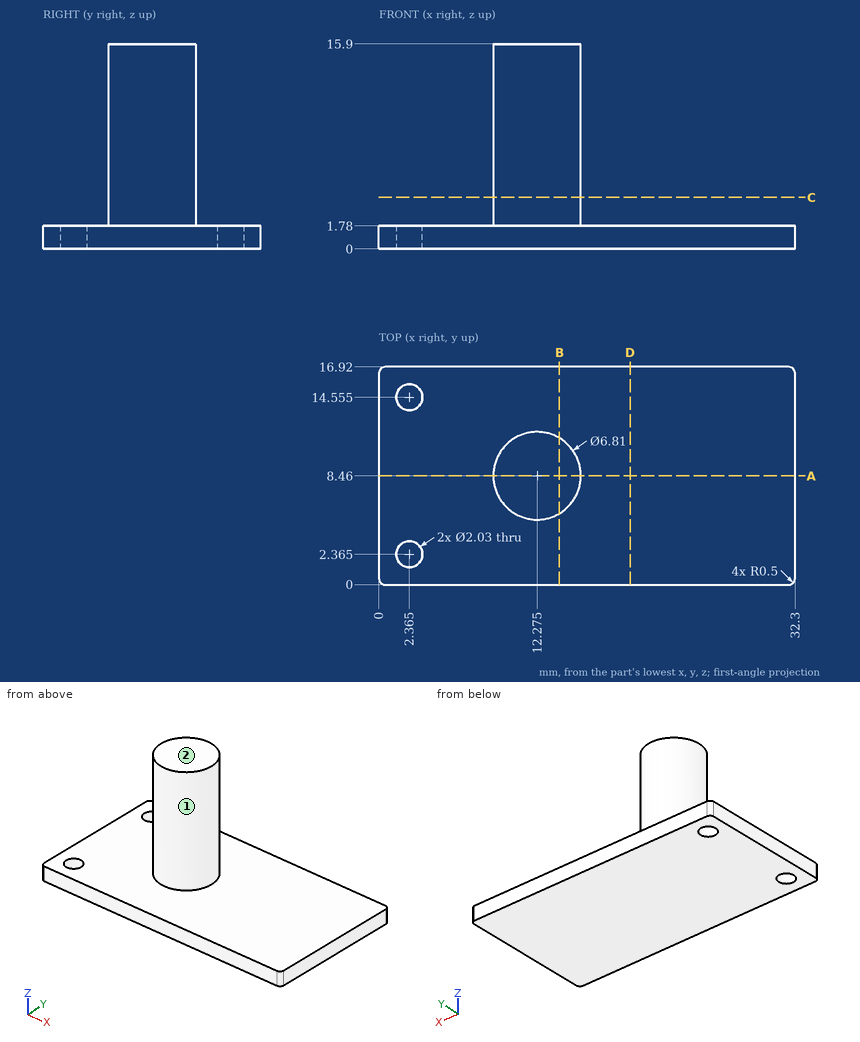
Answer from the drawing. Dimensions are ordinates in mm from the lowest x, y and z of the part. A direction names the side the tool comes from. Give positions to 0.01 mm unless a question says otherwise; leave off trailing zeros. Loops run counter-clockwise (first coordinate to the right, second up) from the corner with the lowest first, then second, coordinate; pieces in that order, holes last. Notation, with made-up numbers: (42.25, 55) - (57.25, 55) arc R25 ccw to (57.25, 78) - close; hole circle Ø8 at (55, 55.5). An arc over 180 degrees is marked (long way). Answer as a JSON object with one key per item and string values.
1. A cutting plane is placed at B-B (x = 14). Write down the section's boundary in (y, z), then the cut area to 3 significant figures.
Determined:
{"outline": "(0, 0) - (16.92, 0) - (16.92, 1.78) - (11.4, 1.78) - (11.4, 15.9) - (5.52, 15.9) - (5.52, 1.78) - (0, 1.78) - close", "area": "113 mm²"}
2. A cutting plane is placed at C-C (z = 4). Write down the section's boundary in (x, y) (3 decimals).
Determined:
{"outline": "circle Ø6.81 at (12.275, 8.46)"}
3. Find the intervals of material crossed by L1, parallel to Z at x = 25.5, y = 4; L2, parallel to Y at x = 9.5, z = 7; L3, parallel to X at y = 8, z = 3.5, in increasing order. Write a range as [from, to].
Determined:
{"L1": "[0, 1.78]", "L2": "[6.49, 10.43]", "L3": "[8.9, 15.65]"}
4. Flat-ended cylindrical pins translate along their axes: pin 1 Ø2 at (x, y) = (24, 11) entering from -Z; pin 2 Ø3 at (x, y) = (22, 6) entering from +Z; pin 3 Ø1.5 at (y, z) = (11, 4.5) entering from -X. Find the tip coordinate at first contact, or state that the pin passes through.
Determined:
{"pin 1": "z = 0", "pin 2": "z = 1.78", "pin 3": "x = 9.38"}
5. A cutting plane is placed at D-D (x = 19.5). Write down the section's boundary in (y, z).
Determined:
{"outline": "(0, 0) - (16.92, 0) - (16.92, 1.78) - (0, 1.78) - close"}
6. For the marked faces 1 and 2, determine the directions among +Z, -Z, +X, -X, +Y, -Y from which every point of the face is accessible in a straight line to the end or side of a thin tool.
Determined:
{"face 1": "+Z", "face 2": "+Z, +X, -X, +Y, -Y"}
7. A cutting plane is placed at A-A (y = 8.46). Write down the section's boundary in (x, z), then the cut area to 3 significant figures.
Determined:
{"outline": "(0, 0) - (32.3, 0) - (32.3, 1.78) - (15.68, 1.78) - (15.68, 15.9) - (8.87, 15.9) - (8.87, 1.78) - (0, 1.78) - close", "area": "154 mm²"}
